Could you check a few things on this model? Use its own coordinates, in mm. A direction names the side the tool comes from. Give positions to 0.01 mm unless a question says otherwise; leave off trailing zeros. Loops run counter-clockwise (first coordinate to the right, second up) from the corner with the lowest first, then second, coordinate; pieces in that order, holes last. Notation, with made-up numbers: (78.5, 58) - (120.5, 58) arc R22 cw to (120.5, 65) - close; hole circle Ø4 at (-19, 1.25). An arc over 180 degrees is marked (long way). Answer in a Markdown table with one row per item. Add a question column.
```python
from build123d import *

# Parameters (mm, degrees)
BOSS_EXTRUDE1_DEPTH = 25
BOSS_EXTRUDE2_DEPTH = 15
SKETCH3_W           = 15
SKETCH3_H           = 15
CUT_EXTRUDE1_DEPTH  = 15


with BuildPart() as part:
    # Sketch1 → Boss-Extrude1 (new body)
    with BuildSketch(Plane.XY):
        Polygon((-30, 10), (-15, 10), (-15, 25), (0, 25), (0, 0), (-30, 0), align=None)
    extrude(amount=BOSS_EXTRUDE1_DEPTH)

    # Sketch2 → Boss-Extrude2 (add)
    with BuildSketch(Plane.ZY.offset(15)):
        Polygon((0, 25), (25, 10), (0, 10), align=None)
    extrude(amount=BOSS_EXTRUDE2_DEPTH)

    # Sketch3 → Cut-Extrude1 (cut)
    with BuildSketch(Plane(origin=(0, 0, 0), x_dir=(-1, 0, 0), z_dir=(0, 0, -1))):
        with Locations((22.5, 7.5)):
            Rectangle(SKETCH3_W, SKETCH3_H)
    extrude(amount=-CUT_EXTRUDE1_DEPTH, mode=Mode.SUBTRACT)


solid = part.part
```
(1) I want a section at A-A on z = 9.25. Please give me the cut outline in (x, y).
(2) On a 3-axis mill with a long thin cutter (end or side, diameter ignored), from which of +Z, -Z, +X, -X, +Y, -Y can I reach the whole of each face in a straight line? I mean faces 1 (the flat face through (-15, 21, 18)), 2 (the flat face through (-11, 0, 15)), 3 (the flat face through (-22, 8, 15)). Say none if no direction works.
(3) I want a section at B-B on y = 2. Please give me the cut outline in (x, z).
(4) I want a section at D-D on z = 5. Please give me the cut outline in (x, y), then the cut area to 3 significant figures.
(5) Please list where these lines run through material, in increasing order: line 1 (X direction, y = 9, z = 14.25); line 2 (Z direction, x = -23, y = 4.5); line 3 (Z direction, x = -25.75, y = 16).
(6) For pin 1 Ø4 at (y, z) = (11, 3) entering from -X, with a flat end and sliding along its axis, tell me the tip position at first contact or that it passes through.
(7) I want a section at C-C on x = -20.75. Please give me the cut outline in (y, z).
Reported:
| question | item | result |
|---|---|---|
| 1 | outline | (-30, 15) - (-15, 15) - (-15, 0) - (0, 0) - (0, 25) - (-15, 25) - (-15, 19.45) - (-30, 19.45) - close |
| 2 | face 1 | +Z, -X, +Y |
| 2 | face 2 | +Z, -Z, +X, -X, -Y |
| 2 | face 3 | -Z, -X, -Y |
| 3 | outline | (-30, 15) - (-15, 15) - (-15, 0) - (0, 0) - (0, 25) - (-30, 25) - close |
| 4 | outline | (-30, 15) - (-15, 15) - (-15, 0) - (0, 0) - (0, 25) - (-15, 25) - (-15, 22) - (-30, 22) - close |
| 4 | area | 480 mm² |
| 5 | line 1 | -15 to 0 |
| 5 | line 2 | 15 to 25 |
| 5 | line 3 | 0 to 15 |
| 6 | pin 1 | x = -15 |
| 7 | outline | (0, 15) - (15, 15) - (15, 0) - (25, 0) - (10, 25) - (0, 25) - close |
